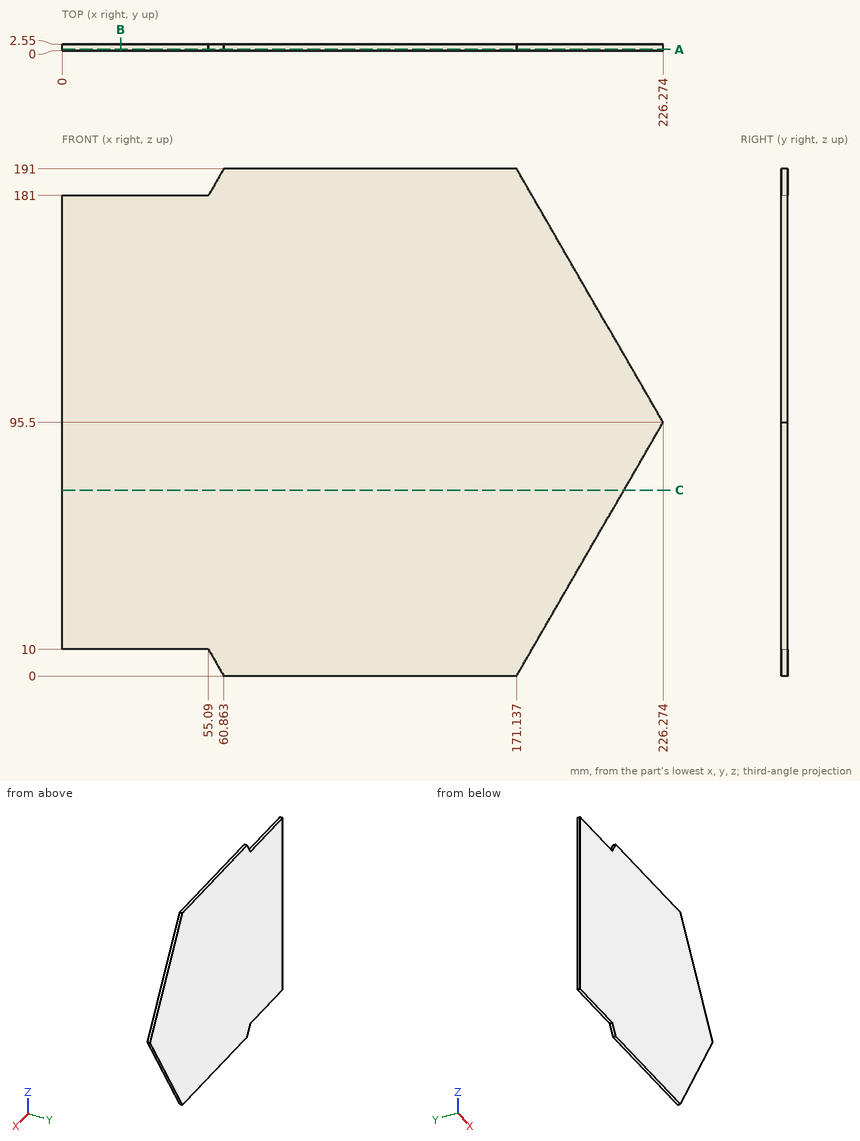
Input: dimensioned drawing with shaded views. Units: mm. Origin: part minimum x, y, z. Give positions to 0.01 mm unless a question says otherwise; leave off trailing zeros. Write each loop counter-clockwise with the first axis right and the second up, starting at its lowest first coordinate (ties: lowest second). Pieces come first, ordered by that corner, then holes.
1. Section query A-A (y = 0.5). Return the cut outline in (x, z), then the cut area to 3 significant figures.
2. Material intervals for line 1 along Z through (x, y) = (44.5, 1.25); line 2 along X through (y, z) = (0.35, 129.5) (1 decimal); line 3 along X through (y, z) = (0.8, 160) (1 decimal), sorted ascending.
3. First-contact query: pin 1 (1.5 mm diameter, centred on y = 1, z = 151, fed in from +X) (1 decimal); pin 2 (1.3 mm diameter, centred on x = 37.5, y = 1, fed in from +Z). Flat tips, straight axial feed; report the tip coordinate or a pass-through.
4. Section query B-B (x = 22). Return the cut outline in (y, z).
5. Section query C-C (z = 70). Return the cut outline in (x, y).
Output values:
1. outline: (0, 10) - (55.09, 10) - (60.86, 0) - (171.14, 0) - (226.27, 95.5) - (171.14, 191) - (60.86, 191) - (55.09, 181) - (0, 181) - close
1. area: 36,800 mm2
2. line 1: z = 10 to 181
2. line 2: x = 0 to 206.6
2. line 3: x = 0 to 189
3. pin 1: stops at x = 194.7
3. pin 2: stops at z = 181
4. outline: (0, 10) - (2.55, 10) - (2.55, 181) - (0, 181) - close
5. outline: (0, 0) - (211.55, 0) - (211.55, 2.55) - (0, 2.55) - close
